The model under review builds one solid part; all positions refer to its coordinate system, in mm. Face numbers are marked on the shaded views. A direction names the side the tool comes from. Round coordinates to 2 decimals unless told otherwise and drop trailing zeros. Loops run counter-clockwise (first coordinate to the right, second up) from the corner with the lowest first, then second, coordinate; pieces in that order, holes last. Notation, with made-up numbers: (-15.75, 7.25) - (27.25, 7.25) arc R20 cw to (27.25, 23.25) - close; hole circle Ø1 at (85, 69). An arc over 180 degrees is marked (long way). Answer as CSV lines item,"result".
from build123d import *

# Parameters (mm, degrees)
SKETCH1_W           = 21
SKETCH1_H           = 48
SKETCH1_R           = 7
BOSS_EXTRUDE1_DEPTH = 5
SKETCH2_W           = 5
SKETCH2_H           = 48
BOSS_EXTRUDE2_DEPTH = 36
SKETCH4_W           = 16
SKETCH4_H           = 5
BOSS_EXTRUDE3_DEPTH = 18
CUT_EXTRUDE1_DEPTH  = 64.568860301
SKETCH6_R           = 2.05
CUT_EXTRUDE2_DEPTH  = 18


with BuildPart() as part:
    # Sketch1 → Boss-Extrude1 (new body)
    with BuildSketch(Plane(origin=(0, 0, 0), x_dir=(1, 0, 0), z_dir=(0, 1, 0))):
        with Locations((10.5, -24)):
            Rectangle(SKETCH1_W, SKETCH1_H)
        with Locations(Location((13, -24, 0), (0, 0, 270))):
            Circle(SKETCH1_R, mode=Mode.SUBTRACT)
    extrude(amount=BOSS_EXTRUDE1_DEPTH)

    # Sketch2 → Boss-Extrude2 (add)
    with BuildSketch(Plane.XZ):
        with Locations((2.5, 24)):
            Rectangle(SKETCH2_W, SKETCH2_H)
    extrude(amount=BOSS_EXTRUDE2_DEPTH)

    # Sketch4 → Boss-Extrude3 (add)
    with BuildSketch(Plane.XZ):
        with Locations((13, 45.5)):
            Rectangle(SKETCH4_W, SKETCH4_H)
        with Locations((13, 2.5)):
            Rectangle(SKETCH4_W, SKETCH4_H)
    extrude(amount=BOSS_EXTRUDE3_DEPTH)

    # Sketch5 → Cut-Extrude1 (cut, through all)
    with BuildSketch(Plane.XY.offset(48)):
        Polygon((21, 0), (5, -18), (21, -18), align=None)
    extrude(amount=-CUT_EXTRUDE1_DEPTH, mode=Mode.SUBTRACT)

    # Sketch6 → Cut-Extrude2 (cut)
    with BuildSketch(Plane.ZY):
        with Locations((8, -31)):
            Circle(SKETCH6_R)
        with Locations((16, -31)):
            Circle(SKETCH6_R)
        with Locations((24, -31)):
            Circle(SKETCH6_R)
        with Locations((32, -31)):
            Circle(SKETCH6_R)
        with Locations((40, -31)):
            Circle(SKETCH6_R)
        with Locations((16, -23)):
            Circle(SKETCH6_R)
        with Locations((24, -23)):
            Circle(SKETCH6_R)
        with Locations((32, -23)):
            Circle(SKETCH6_R)
        with Locations((40, -23)):
            Circle(SKETCH6_R)
        with Locations((16, -15)):
            Circle(SKETCH6_R)
        with Locations((24, -15)):
            Circle(SKETCH6_R)
        with Locations((32, -15)):
            Circle(SKETCH6_R)
        with Locations((40, -15)):
            Circle(SKETCH6_R)
        with Locations((8, -23)):
            Circle(SKETCH6_R)
        with Locations((8, -15)):
            Circle(SKETCH6_R)
    extrude(amount=-CUT_EXTRUDE2_DEPTH, mode=Mode.SUBTRACT)


solid = part.part
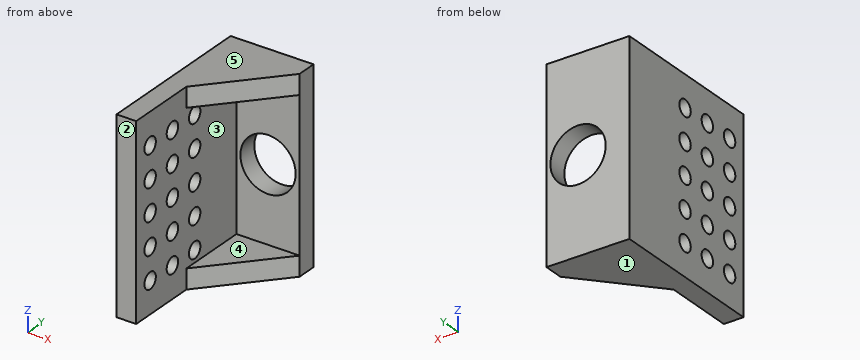
1. Take a section at C-C (x = 3.25). State how many separate pieces and enclosed holes the cut face has, plus the area to 3 significant figures.
Numbers:
separate pieces,"1"
enclosed holes,"15"
area,"1,770 mm²"
2. Take a section at B-B (z = 32). State the section outline as (x, y) points.
Numbers:
outline,"(0, -36) - (5, -36) - (5, -33.05) - (0, -33.05) - close; (0, -28.95) - (5, -28.95) - (5, -25.05) - (0, -25.05) - close; (0, -20.95) - (5, -20.95) - (5, -17.05) - (0, -17.05) - close; (0, -12.95) - (5, -12.95) - (5, 0) - (21, 0) - (21, 5) - (0, 5) - close"
3. Draft analysis for pull direction Z (two halves, no side actions). For the marked faces 1, 2 and 3, state which applies: +Z half, -Z half, draft (parallel to the pull), parting line (faces both ways), or undercut.
Numbers:
face 1,"-Z half"
face 2,"draft"
face 3,"undercut"
4. Tool access review of the marked faces 4 and 5: name each direction out of +Z, -Z, +X, -X, +Y, -Y from which nothing blocks a thin tool from reaching the whole face with its end or side.
Numbers:
face 4,"+X, -Y"
face 5,"+Z, +X, -X, +Y, -Y"
5. Clearance check with flat-ended pins moving along their axes: pin 1 (12 mm diameter, centred on y = -22.5, z = 12.5, fed in from +X); pin 2 (6 mm diameter, centred on x = 9, z = 20.5, fed in from -Y). State where each tip first meets the part, or that it passes through.
Numbers:
pin 1,"stops at x = 5"
pin 2,"stops at y = 0"
6. Wall thickness on probe 1 along Y at (x, z) = (3.5, 40); probe 2 along Z at (x, y) = (5.5, -5); probe 3 along X at (y, z) = (1.75, 24): over which ranges is each line inside the solid? List them lowest first.
Numbers:
probe 1,"y = -36 to -33.05, -28.95 to -25.05, -20.95 to -17.05, -12.95 to 5"
probe 2,"z = 0 to 5, 43 to 48"
probe 3,"x = 0 to 6, 20 to 21"
7. Take a section at D-D (y = -31). State the section outline as (x, z) points.
Numbers:
outline,"(0, 0) - (5, 0) - (5, 5.95) - (0, 5.95) - close; (0, 10.05) - (5, 10.05) - (5, 13.95) - (0, 13.95) - close; (0, 18.05) - (5, 18.05) - (5, 21.95) - (0, 21.95) - close; (0, 26.05) - (5, 26.05) - (5, 29.95) - (0, 29.95) - close; (0, 34.05) - (5, 34.05) - (5, 37.95) - (0, 37.95) - close; (0, 42.05) - (5, 42.05) - (5, 48) - (0, 48) - close"
8. Take a section at A-A (z = 24). State the section outline as (x, y) points.
Numbers:
outline,"(0, -36) - (5, -36) - (5, -33.05) - (0, -33.05) - close; (0, -28.95) - (5, -28.95) - (5, -25.05) - (0, -25.05) - close; (0, -20.95) - (5, -20.95) - (5, -17.05) - (0, -17.05) - close; (0, -12.95) - (5, -12.95) - (5, 0) - (6, 0) - (6, 5) - (0, 5) - close; (20, 0) - (21, 0) - (21, 5) - (20, 5) - close"
